Geometry: final body of the model. Coordinates: model frame, mm. A direction names the side the tool comes from. Coordinates: 2 decimals unless noted, no trailing zeros. Order: outer loops, then holes, each group sorted by start corner. A loop starts at its lowest first (then second) coordinate and runs counter-clockwise, first axis right, second up. Notation, with made-up numbers: (58.25, -30.5) - (98.25, -30.5) arc R19 cw to (98.25, 4.5) - close; hole circle Ø7 at (0.25, 29). An arc over 180 degrees is marked (long way). Use a Markdown table: item, result. Add a question column.
```python
from build123d import *

# Parameters (mm, degrees)
SKETCH1_R               = 30
BOSS_EXTRUDE1_DEPTH     = 10
SKETCH2_R               = 10
SKETCH2_R_2             = 4
BOSS_EXTRUDE2_DEPTH     = 10
CUT_EXTRUDE1_DEPTH      = 10
CUT_EXTRUDE1_DEPTH_BACK = 10
SKETCH3_R               = 2


with BuildPart() as part:
    # Sketch1 → Boss-Extrude1 (new body)
    with BuildSketch(Plane.XY):
        Circle(SKETCH1_R)
    extrude(amount=BOSS_EXTRUDE1_DEPTH)

    # Sketch2 → Boss-Extrude2 (add)
    with BuildSketch(Plane.XY.offset(10)):
        Circle(SKETCH2_R)
        Circle(SKETCH2_R_2, mode=Mode.SUBTRACT)
    extrude(amount=BOSS_EXTRUDE2_DEPTH)

    # Sketch3 → Cut-Extrude1 (cut, two sides: drawn at the far end of the back side and taken through both)
    with BuildSketch(Plane(origin=(0, 0, 0), x_dir=(0, 0, -1), z_dir=(1, 0, 0)).offset(-CUT_EXTRUDE1_DEPTH_BACK)):
        with Locations(Location((-15, 0, 0), (0, 0, 180))):
            Circle(SKETCH3_R)
    extrude(amount=CUT_EXTRUDE1_DEPTH + CUT_EXTRUDE1_DEPTH_BACK, mode=Mode.SUBTRACT)


solid = part.part
```
1) Section D-D (z = 5). Return loops of the section in (x, y).
2) Pin query (flat end, axial travel): pin 1 (6.5 mm diameter, centred on y = 0, z = 15, fed in from -X); pin 2 (4 mm diameter, centred on x = -6, y = -2.5, fed in from -Z); pin 3 (1.5 mm diameter, centred on x = 9.5, z = 4, fed in from +Y); pin 4 (6 mm diameter, centred on x = -17.5, z = 9.5, fed in from +Y). Return the tip coordinate at first contact, or that it passes through.
3) Draft query along Z for faces 1 (the face through (0, 0, 10)), 2 (the face through (-7, 0, 13)), 3 (the face through (-29.97, 1.32, 4.93)), 4 (the face through (7, -2, 15)). Return one class per face: pulls with the +Z half, pulls with the -Z half, needs draft (parallel to the pull), parting line crosses it, or undercut.
4) Ray query, line 1 along Y through (x, z) = (0, 13.25); line 2 along Z through (x, y) = (-9.5, 16); line 3 along Y through (x, z) = (6.75, 15). Return the intervals inside material, ascending.
5) Section C-C (z = 15.5). Return loops of the section in (x, y).
6) Section B-B (x = 0). Return loops of the section in (y, z), then the cut area to 3 significant figures.
7) Section A-A (y = 0). Return loops of the section in (x, z), then the cut area to 3 significant figures.
8) Set-up query: faces 5 (the face through (-0.1, -4.3, 20)), 6 (the face through (9.54, 3, 14.93)). Return all of +Z, -Z, +X, -X, +Y, -Y with unobstructed straight access to the full face (end or side cutting, diameter ignored); none if empty.
Values follow:
| question | item | result |
|---|---|---|
| 1 | outline | circle Ø60 at (0, 0) |
| 2 | pin 1 | stops at x = -10 |
| 2 | pin 2 | stops at z = 0 |
| 2 | pin 3 | stops at y = 28.7 |
| 2 | pin 4 | stops at y = 26.26 |
| 3 | face 1 | pulls with the +Z half |
| 3 | face 2 | undercut |
| 3 | face 3 | needs draft |
| 3 | face 4 | undercut |
| 4 | line 1 | y = -10 to -4, 4 to 10 |
| 4 | line 2 | z = 0 to 10 |
| 4 | line 3 | y = -7.38 to -2, 2 to 7.38 |
| 5 | outline | (-9.81, -1.94) arc R10 ccw to (9.81, -1.94) - (3.5, -1.94) arc R4 cw to (-3.5, -1.94) - close; (-9.81, 1.94) - (-3.5, 1.94) arc R4 cw to (3.5, 1.94) - (9.81, 1.94) arc R10 ccw to start |
| 6 | outline | (-30, 0) - (30, 0) - (30, 10) - (10, 10) - (10, 20) - (4, 20) - (4, 10) - (-4, 10) - (-4, 20) - (-10, 20) - (-10, 10) - (-30, 10) - close |
| 6 | area | 720 mm² |
| 7 | outline | (-30, 0) - (30, 0) - (30, 10) - (10, 10) - (10, 13) - (4, 13) - (4, 10) - (-4, 10) - (-4, 13) - (-10, 13) - (-10, 10) - (-30, 10) - close; (-10, 17) - (-4, 17) - (-4, 20) - (-10, 20) - close; (4, 17) - (10, 17) - (10, 20) - (4, 20) - close |
| 7 | area | 672 mm² |
| 8 | face 5 | +Z, +X, -X, +Y, -Y |
| 8 | face 6 | +Z |
